Part model, mm, in its own coordinate system. Face numbers are marked on the shaded views. A direction names the side the tool comes from. Give positions to 0.01 mm unless a question says otherwise; leave off trailing zeros. Write each loop counter-clockwise with the first axis right and the second up, starting at its lowest first coordinate (ties: lowest second). Pieces come first, ordered by that corner, then holes. Notation, with made-up numbers: M 25,1.25 L 78,1.25 A15 ccw 78,7.25 Z; hole C 4,61 d2. An arc over 180 degrees is marked long. Answer as CSV lines item,"result". Start each with the question number.
1) Slice it at A-A, the plane z = 103. Give the cut face in (x, y).
2) Pin check, flat tips, straight feed: pin 1 Ø12 at (x, y) = (-360, 225) entering from -Z; pin 2 Ø6 at (x, z) = (-99, 30.5) entering from +Y; pin 3 Ø5 at (y, z) = (93, -123.5) entering from +X. Stop position of each tip, or through.
3) Wall check: line 1 along Z through (x, y) = (-120, 44.5); line 2 along Z through (x, y) = (-293, 93); line 3 along X through (y, z) = (135, -56.5). Give the ranges that are in metal, low to high. Write a range as from..to.
4) Slice it at B-B, the plane x = 73.5. Give the cut face in (y, z).
5) Slice it at D-D, the plane z = 0. Give the cut face in (x, y), plus the area to 3 significant figures.
6) Mould opens along X. For the marked faces 1, 2, 3 and 4 say: pulls with the +X half, pulls with the -X half, needs draft (parallel to the pull), parting line crosses it, or undercut.
7) Tool access for the marked faces 5, 6 and 7: list every direction of +Z, -Z, +X, -X, +Y, -Y with a clear straight run to the whole face (end or side of a thin tool).
8) Slice it at C-C, the plane x = 240. Give the cut face in (y, z).
```python
from build123d import *

# Parameters (mm, degrees)
SKETCH_1_W              = 770
SKETCH_1_H              = 360
SKETCH_1_W_2            = 670
SKETCH_1_H_2            = 260
EXTRUDE_1_DEPTH         = 50
SKETCH_2_R              = 10
EXTRUDE_2_DEPTH         = 50
SKETCH_3_R              = 10
EXTRUDE_3_DEPTH         = 50
SKETCH_4_W              = 670
SKETCH_4_H              = 80
EXTRUDE_4_DEPTH         = 50
SKETCH_8_W              = 50
SKETCH_8_H              = 260
EXTRUDE_6_DEPTH         = 100
PATTERN_LINEAR_27_COUNT = 3
PATTERN_LINEAR_27_PITCH = 120
SKETCH_12_W             = 50
SKETCH_12_H             = 260
EXTRUDE_10_DEPTH        = 50
FILLET_3_R              = 10


with BuildPart() as part:
    # 草图1 → 凸台-拉伸1 (new body)
    with BuildSketch(Plane(origin=(0, 0, 0), x_dir=(1, 0, 0), z_dir=(0, 1, 0))):
        Rectangle(SKETCH_1_W, SKETCH_1_H)
        Rectangle(SKETCH_1_W_2, SKETCH_1_H_2, mode=Mode.SUBTRACT)
    extrude(amount=EXTRUDE_1_DEPTH)

    # 草图2 → 凸台-拉伸2 (add)
    with BuildSketch(Plane.XY.offset(180)):
        with BuildLine():
            Line((-385, 50), (-385, 225))
            ThreePointArc((-385, 225), (-369.567085809, 248.096988313), (-342.32233047, 242.67766953))
            Line((-342.32233047, 242.67766953), (-149.644660941, 50))
            Line((-149.644660941, 50), (-385, 50))
        make_face()
        with Locations((-360, 225)):
            Circle(SKETCH_2_R, mode=Mode.SUBTRACT)
    extrude(amount=-EXTRUDE_2_DEPTH)

    # 草图3 → 凸台-拉伸3 (add)
    with BuildSketch(Plane(origin=(0, 0, -180), x_dir=(-1, 0, 0), z_dir=(0, 0, -1))):
        with BuildLine():
            Line((149.644660941, 50), (385, 50))
            Line((385, 50), (385, 225))
            ThreePointArc((385, 225), (369.567085809, 248.096988313), (342.32233047, 242.67766953))
            Line((342.32233047, 242.67766953), (149.644660941, 50))
        make_face()
        with Locations((360, 225)):
            Circle(SKETCH_3_R, mode=Mode.SUBTRACT)
    extrude(amount=-EXTRUDE_3_DEPTH)

    # 草图4 → 凸台-拉伸4 (add)
    with BuildSketch(Plane(origin=(0, 50, 0), x_dir=(1, 0, 0), z_dir=(0, 1, 0))):
        Rectangle(SKETCH_4_W, SKETCH_4_H)
    extrude(amount=-EXTRUDE_4_DEPTH)

    # 草图8 → 凸台-拉伸6 (add)
    with BuildSketch(Plane(origin=(0, 50, 0), x_dir=(1, 0, 0), z_dir=(0, 1, 0))):
        with Locations((-360, 0)):
            Rectangle(SKETCH_8_W, SKETCH_8_H)
    extrude(amount=EXTRUDE_6_DEPTH)

    # 草图11 → 旋转1 (revolve)
    with BuildSketch(Plane.XY):
        with BuildLine():
            Line((0, 50), (12.5, 50))
            Line((12.5, 50), (12.5, 53.349364905))
            ThreePointArc((12.5, 53.349364905), (24.148145657, 81.470476128), (0, 100))
            Line((0, 100), (0, 99.72990561))
            Line((0, 99.72990561), (0, 50))
        make_face()
    revolve_1 = revolve(axis=Axis((0, 50, 0), (0, 1, 0)))

    # 阵列(线性)27: 旋转1 ×3
    with Locations(*[(i * PATTERN_LINEAR_27_PITCH, 0, 0) for i in range(1, PATTERN_LINEAR_27_COUNT)]):
        add(revolve_1)

    # 草图12 → 凸台-拉伸10 (add)
    with BuildSketch(Plane(origin=(0, 50, 0), x_dir=(1, 0, 0), z_dir=(0, 1, 0))):
        Rectangle(SKETCH_12_W, SKETCH_12_H)
        with Locations((120, 0)):
            Rectangle(SKETCH_12_W, SKETCH_12_H)
        with Locations((240, 0)):
            Rectangle(SKETCH_12_W, SKETCH_12_H)
    extrude(amount=-EXTRUDE_10_DEPTH)

    # 圆角3
    fillet_3_edges = [part.edges().sort_by_distance(p)[0] for p in [
        (-25, 25, 40),
        (25, 25, 40),
        (25, 25, -40),
        (25, 25, -130),
        (-25, 25, -40),
        (25, 25, 130),
        (-25, 25, 130),
        (-25, 25, -130),
        (145, 25, -40),
        (145, 25, -130),
        (95, 25, -40),
        (95, 25, -130),
        (145, 25, 40),
        (145, 25, 130),
        (95, 25, 40),
        (95, 25, 130),
        (-335, 75, 130),
        (335, 25, 130),
        (335, 25, -130),
        (-335, 75, -130),
        (265, 25, -40),
        (265, 25, -130),
        (215, 25, -40),
        (215, 25, -130),
        (265, 25, 40),
        (265, 25, 130),
        (215, 25, 40),
        (215, 25, 130),
        (-245.983495706, 146.338834765, 180),
        (-369.567085809, 248.096988313, 180),
        (-245.983495706, 146.338834765, -180),
        (-369.567085809, 248.096988313, -180),
        (-335, 25, 40),
        (-335, 25, -40),
        (335, 25, -40),
        (335, 25, 40),
        (-385, 112.5, -180),
        (385, 25, -180),
        (385, 25, 180),
        (-385, 112.5, 180),
    ]]
    fillet(fillet_3_edges, radius=FILLET_3_R)


solid = part.part
```
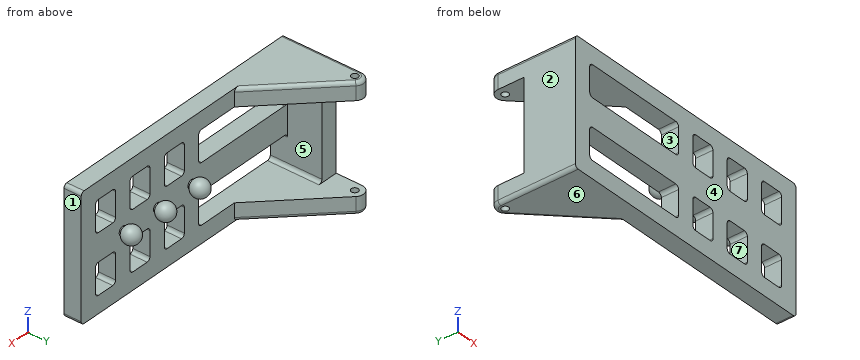
Found:
1,outline,"M -385,0 L -335,0 L -335,150 L -385,150 Z; M -25,0 L 25,0 L 25,50 L -25,50 Z; M 95,0 L 145,0 L 145,50 L 95,50 Z; M 215,0 L 265,0 L 265,50 L 215,50 Z; M 335,0 L 385,0 L 385,50 L 335,50 Z"
2,pin 1,"through"
2,pin 2,"y = 50"
2,pin 3,"x = -333"
3,line 1,"-180..-130, -40..40, 130..180"
3,line 2,"-180..-130, 130..180"
3,line 3,"-385..-335"
4,outline,"M 0,-180 L 50,-180 L 50,-130 L 0,-130 Z; M 0,-40 L 50,-40 L 50,40 L 0,40 Z; M 0,130 L 50,130 L 50,180 L 0,180 Z"
5,outline,"M -385,0 L 385,0 L 385,50 L 252.5,50 L 252.5,53.35 A25 ccw long 227.5,53.35 L 227.5,50 L 132.5,50 L 132.5,53.35 A25 ccw long 107.5,53.35 L 107.5,50 L 12.5,50 L 12.5,53.35 A25 ccw long -12.5,53.35 L -12.5,50 L -335,50 L -335,150 L -385,150 Z"
5,area,"49,500 mm²"
6,face 1,"pulls with the +X half"
6,face 2,"pulls with the -X half"
6,face 3,"undercut"
6,face 4,"needs draft"
7,face 5,"+Y"
7,face 6,"-Z, +X, -X, +Y, -Y"
7,face 7,"+Y, -Y"
8,outline,"M 0,-180 L 50,-180 L 50,-12.5 L 53.35,-12.5 A25 ccw long 53.35,12.5 L 50,12.5 L 50,180 L 0,180 Z"
